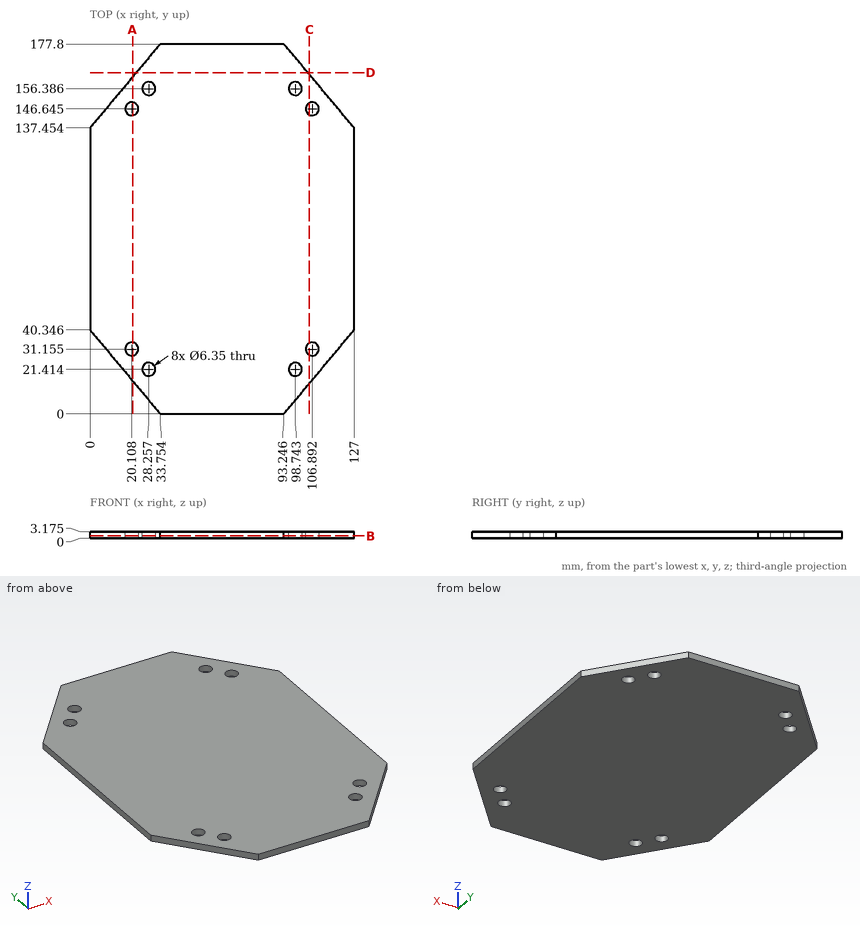
Geometry check sheet. Reference: drawing and pictorial views, mm from the part's lowest x, y, z. Coordinates: 2 decimals unless noted, no trailing zeros. Write each loop counter-clockwise with the first axis right and the second up, starting at its lowest first coordinate (ties: lowest second). Pieces come first, ordered by that corner, then holes. Notation, with made-up numbers: M -29.5,25 L 6.5,25 A20 ccw 6.5,47 Z; hole C -17.75,18.25 d9. An arc over 180 degrees is marked long. One line per question, with ' | ' between items.
1) Sectioned sample at A-A on x = 20.5. Record the cut outline in (y, z) (1 decimal), then the cut area to 3 significant figures.
Solutions:
outline: M 15.8,0 L 28,0 L 28,3.2 L 15.8,3.2 Z; M 34.3,0 L 143.5,0 L 143.5,3.2 L 34.3,3.2 Z; M 149.8,0 L 162,0 L 162,3.2 L 149.8,3.2 Z | area: 424 mm^2
2) Sectioned sample at B-B on z = 1.2. State how many separate pieces and enclosed holes the cut face has, then the cut area to 3 significant figures.
Solutions:
separate pieces: 1 | enclosed holes: 8 | area: 19,600 mm^2
3) Sectioned sample at C-C on x = 105.5. Record the cut outline in (y, z) (1 decimal).
Solutions:
outline: M 14.6,0 L 28.3,0 L 28.3,3.2 L 14.6,3.2 Z; M 34,0 L 143.8,0 L 143.8,3.2 L 34,3.2 Z; M 149.5,0 L 163.2,0 L 163.2,3.2 L 149.5,3.2 Z
4) Material ranges on L1, parallel to Y at x = 30, z = 0.35 (1 decimal); L2, parallel to Y at x = 26.5, z = 1.7; L3, parallel to Y at x = 115.5, z = 2.4, recorded low to high.
Solutions:
L1: 4.5 to 18.8, 24.1 to 153.7, 159 to 173.3 | L2: 8.67 to 18.77, 24.06 to 153.74, 159.03 to 169.13 | L3: 26.6 to 151.2
5) Sectioned sample at D-D on y = 164. Record the cut outline in (x, z) (1 decimal).
Solutions:
outline: M 22.2,0 L 104.8,0 L 104.8,3.2 L 22.2,3.2 Z
